```python
from build123d import *

# Parameters (mm, degrees)
SKETCH2_R           = 1
BOSS_EXTRUDE1_DEPTH = 1
SKETCH3_W           = 2
SKETCH3_H           = 1
CUT_EXTRUDE1_DEPTH  = 5


with BuildPart() as part:
    # Sketch1 → Revolve1 (revolve)
    with BuildSketch(Plane.XY):
        with BuildLine():
            Line((0, 5), (0, -5))
            Line((0, -5), (2, -5))
            Line((2, -5), (2, -4))
            Line((2, -4), (3.33, -4))
            Line((3.33, -4), (3.33, 3))
            Line((3.33, 3), (5, 3))
            Line((5, 3), (5, 5))
            ThreePointArc((5, 5), (3.168263504, 6.198702678), (1, 6.5))
            Line((1, 6.5), (1, 5.5))
            Line((1, 5.5), (0, 5.5))
            Line((0, 5.5), (0, 5))
        make_face()
    revolve(axis=Axis((0, 5, 0), (0, -1, 0)))

    # Sketch2 → Boss-Extrude1 (add)
    with BuildSketch(Plane(origin=(0, 5.5, 0), x_dir=(1, 0, 0), z_dir=(0, 1, 0))):
        Circle(SKETCH2_R)
    extrude(amount=BOSS_EXTRUDE1_DEPTH)

    # Sketch3 → Cut-Extrude1 (cut, symmetric)
    with BuildSketch(Plane.XY):
        with Locations((0, 6.01705679)):
            Rectangle(SKETCH3_W, SKETCH3_H)
    extrude(amount=CUT_EXTRUDE1_DEPTH, both=True, mode=Mode.SUBTRACT)


solid = part.part
```
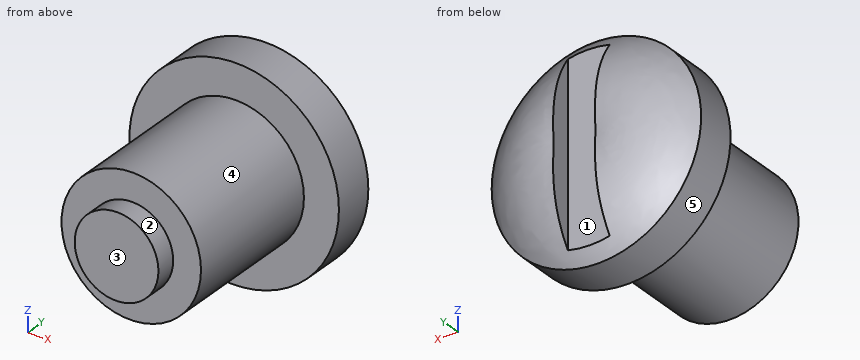
Build history of the part. All positions in model axes, mm. Face numbers are marked on the shaded views. A direction names the side the tool comes from. Round coordinates to 2 decimals unless told otherwise and drop trailing zeros. Write each loop counter-clockwise with the first axis right and the second up, starting at its lowest first coordinate (ties: lowest second). Pieces come first, ordered by that corner, then holes.
1) 3-axis set-ups, long thin cutter, end or side, ignore diameter. For the marked faces 4 and 5: which of +Z, -Z, +X, -X, +Y, -Y reach the whole face in a straight line?
2) Mould opens along X. For the marked faces 1, 2 and 3 say: +X half, -X half, draft (parallel to the pull), parting line (faces both ways), or undercut.
3) Band-saw the part on A-A, the plane y = 0.5. List the corners of the cut face in (x, z).
4) Pin check, flat tips, straight feed: pin 1 (2 mm diameter, centred on y = 3, z = 2.5, fed in from -X); pin 2 (0.6 mm diameter, centred on x = 0, z = 0, fed in from +Y); pin 3 (2 mm diameter, centred on y = -3, z = 0, fed in from -X). Stop position of each tip, or through.
5) Drill centre lines: probe 1 along Z at (x, y) = (-1, 2); probe 2 along Z at (x, y) = (-0.5, 2.5); probe 3 along X at (y, z) = (2, -2). Where is each one in solid material? Low to high.
Ans:
1. face 4: -Y
1. face 5: +Y, -Y
2. face 1: undercut
2. face 2: parting line
2. face 3: draft
3. outline: circle Ø6.66 at (0, 0)
4. pin 1: stops at x = -4.77
4. pin 2: stops at y = 5.52
4. pin 3: stops at x = -3.33
5. probe 1: z = -3.18 to 3.18
5. probe 2: z = -3.29 to 3.29
5. probe 3: x = -2.66 to 2.66
